Read the model definition and answer for the solid it produces. Units are mm, in the model's axes. A direction names the side the tool comes from. Coordinates: 2 decimals unless noted, no trailing zeros. Write each loop counter-clockwise with the first axis right and the second up, starting at its lowest first coordinate (ties: lowest second). Pieces come first, ordered by that corner, then holes.
1) Each of these flat-tipped pins is pushed along its axis until it touches: pin 1 Ø4 at (x, y) = (-14.5, 35.5) entering from +Z; pin 2 Ø12 at (y, z) = (31.5, 43) entering from +X; pin 3 Ø1.5 at (x, z) = (19.5, 11.5) entering from +Y. Where does it stop, or does it pass through?
2) Which of the six approach directions +Z, -Z, +X, -X, +Y, -Y give full straight-line access (tool end or side, diameter ignored) to faces 5 (the face through (-18.807, 29.509, 29.502)), 6 (the face through (2.37, 36.92, 11.14))?
3) The part is cut by section A-A (z = 5.5). Determine the outline of the cut face in (x, y), then the cut area to 3 significant figures.
4) Determine the mould class of faces 1 (the face through (19.189, 30.025, 29.502)), 2 (the face through (2, 37.82, 4)), 3 (the face through (-25.539, 19.323, 4.563)), 4 (the face through (29.529, 19.245, 4.563)) for opening direction X: +X half, -X half, draft (parallel to the pull), parting line (faces both ways), or undercut.
5) The part is cut by section D-D (z = 43.5). Determine the outline of the cut face in (x, y).
6) The part is cut by section B-B (x = -2.5). Determine the outline of the cut face in (y, z), then the cut area to 3 significant figures.
7) Find the intervals of material crossed by line 1 (Z direction, x = 26.5, y = 25.25); line 2 (X direction, y = 29, z = 42); line 3 (X direction, y = 26.5, z = 27), in increasing order.
8) The part is cut by section C-C (y = 31.5). Determine the outline of the cut face in (x, z), then the cut area to 3 significant figures.
from build123d import *

# Parameters (mm, degrees)
F0_W     = 57.996501
F0_H     = 20
F0_R     = 2.5
F1_DEPTH = 12
F2_DEPTH = 50
F3_R     = 2.5
F4_R     = 5
F5_R     = 3


with BuildPart() as f1:
    # F0 (on Top) → F1 (new body)
    with BuildSketch(Plane.XY):
        with Locations((2.033807, 27.819562)):
            Rectangle(F0_W, F0_H)
        with Locations((-16.964443, 27.819562)):
            Circle(F0_R, mode=Mode.SUBTRACT)
        with Locations((21.032058, 28.33525)):
            Circle(F0_R, mode=Mode.SUBTRACT)
        with Locations((-16.964443, 27.819562)):
            Circle(F0_R)
        with Locations((21.032058, 28.33525)):
            Circle(F0_R)
    extrude(amount=F1_DEPTH)

    # F0 (on Top) → F2 (join)
    with BuildSketch(Plane.XY):
        with Locations((-16.964443, 27.819562)):
            Circle(F0_R)
        with Locations((21.032058, 28.33525)):
            Circle(F0_R)
    extrude(amount=F2_DEPTH)

    # F3
    f3_edges = [f1.edges().sort_by_distance(p)[0] for p in [
        (-19.464443, 27.819562, 50),
        (18.532058, 28.33525, 50),
    ]]
    fillet(f3_edges, radius=F3_R)

    # F4
    f4_edges = [f1.edges().sort_by_distance(p)[0] for p in [
        (-26.964443, 37.819562, 6),
        (-26.964443, 17.819562, 6),
        (31.032058, 17.819562, 6),
        (31.032058, 37.819562, 6),
    ]]
    fillet(f4_edges, radius=F4_R)

    # F5
    f5_edges = [f1.edges().sort_by_distance(p)[0] for p in [
        (2.033808, 37.819562, 12),
    ]]
    fillet(f5_edges, radius=F5_R)


solid = f1.part
Reported:
1. pin 1: stops at z = 12
1. pin 2: stops at x = 23.53
1. pin 3: stops at y = 37.26
2. face 5: +Z
2. face 6: +Z, +X, -X, +Y
3. outline: (-26.96, 22.82) arc R5 ccw to (-21.96, 17.82) - (26.03, 17.82) arc R5 ccw to (31.03, 22.82) - (31.03, 32.82) arc R5 ccw to (26.03, 37.82) - (-21.96, 37.82) arc R5 ccw to (-26.96, 32.82) - close
3. area: 1,140 mm2
4. face 1: undercut
4. face 2: draft
4. face 3: -X half
4. face 4: +X half
5. outline: circle Ø5 at (-16.96, 27.82); circle Ø5 at (21.03, 28.34)
6. outline: (17.82, 0) - (37.82, 0) - (37.82, 9) arc R3 ccw to (34.82, 12) - (20.82, 12) arc R3 ccw to (17.82, 9) - close
6. area: 236 mm2
7. line 1: z = 0 to 12
7. line 2: x = -19.17 to -14.76, 18.62 to 23.44
7. line 3: x = -19.09 to -14.84, 19.33 to 22.73
8. outline: (-26.96, 0) - (31.03, 0) - (31.03, 9) arc R3 ccw to (28.03, 12) - (-23.96, 12) arc R3 ccw to (-26.96, 9) - close
8. area: 692 mm2
